Design review of the part built by this model. Coordinates are the model's own, in mm. A direction names the side the tool comes from. Coordinates: 2 decimals unless noted, no trailing zeros. Loops run counter-clockwise (first coordinate to the right, second up) from the corner with the lowest first, then second, coordinate; pieces in that order, holes last.
Q1. Add section B-B on x = -106. Give the boundary of the cut face in (y, z).
Q2. Wall thickness on probe 1 along Z at (x, y) = (-49.5, 190.5); probe 2 along X at (y, z) = (197.5, 81); probe 3 along Z at (x, y) = (-186, 47): over which ranges is each line inside the solid? List them lowest first.
Q3. Add section D-D on y = 19. Give the boundary of the cut face in (x, z).
Q4. Draft analysis for pull direction Y (two halves, no side actions). For faces 5 (the face through (-55.72, 55.49, -4.93)), 6 (the face through (-99, 120, -10)), 7 (the face through (-2.85, 232.99, -22.32)), 8 (the face through (-196.99, 2.85, -22.68)), state which applies: released by +Y, released by -Y, zero draft, split by the parting line, or undercut.
Q5. Add section A-A on y = 190.5. Give the boundary of the cut face in (x, z).
Q6. Machinability: for faces 1 (the face through (-30, 30, 0)), 2 (the face through (-64, 198, 7)), 3 (the face through (-60, 22, -5)), 4 (the face through (-22, 60, -5)), which of the approach directions +Z, -Z, +X, -X, +Y, -Y give a long, thin tool a straight path to every point of the face, cutting with its end or side? Answer none if there is none.
Q7. For P1, Ø3, axis at x = -27, z = -4, coming from the +Y side; P2, Ø8, axis at x = -129, y = 62.5, coming from the +Z side; P3, Ø12, axis at x = -25.5, z = 72, coming from the -Y side, all flat-tipped, find the tip position at first contact; note any pin that passes through.
Q8. Add section C-C on z = 73.5. Give the boundary of the cut face in (x, y), and give its area (3 significant figures).
```python
from build123d import *

# Parameters (mm, degrees)
F1_DEPTH = 200
F0_W     = 60
F0_H     = 10
F2_DEPTH = 60
F0_R     = 20.5
F3_DEPTH = 130
F4_R     = 10
F5_R     = 15


with BuildPart() as f1:
    # F0 (on Right) → F1 (new body)
    with BuildSketch(Plane.YZ):
        Polygon((60, -10), (0, -10), (0, -35), (236, -35), (236, -10), (198, -10), (183, -10), align=None)
    extrude(amount=-F1_DEPTH)

    # F0 (on Right) → F2 (join)
    with BuildSketch(Plane.YZ):
        with Locations((30, -5)):
            Rectangle(F0_W, F0_H)
    extrude(amount=-F2_DEPTH)

    # F0 (on Right) → F3 (join)
    with BuildSketch(Plane.YZ):
        with BuildLine():
            ThreePointArc((226, 60), (168.206503, 87.62698), (183, 25.301297))
            ThreePointArc((183, 25.301297), (190.5, 24.5), (198, 25.301297))
            ThreePointArc((198, 25.301297), (218.12698, 37.706503), (226, 60))
        make_face()
        with Locations((190.5, 60)):
            Circle(F0_R, mode=Mode.SUBTRACT)
        with BuildLine():
            Line((183, 25.301297), (183, -10))
            Line((183, -10), (198, -10))
            Line((198, -10), (198, 25.301297))
            ThreePointArc((198, 25.301297), (190.5, 24.5), (183, 25.301297))
        make_face()
    extrude(amount=-F3_DEPTH)

    # F4
    f4_edges = [f1.edges().sort_by_distance(p)[0] for p in [
        (0, 0, -17.5),
        (-200, 0, -22.5),
        (0, 236, -22.5),
        (-200, 236, -22.5),
    ]]
    fillet(f4_edges, radius=F4_R)

    # F5
    f5_edges = [f1.edges().sort_by_distance(p)[0] for p in [
        (-60, 60, -5),
    ]]
    fillet(f5_edges, radius=F5_R)


solid = f1.part
```
Entries:
1. outline: (0, -35) - (236, -35) - (236, -10) - (198, -10) - (198, 25.3) arc R35.5 ccw to (226, 60) arc R35.5 ccw (long way) to (183, 25.3) - (183, -10) - (0, -10) - close; hole circle Ø41 at (190.5, 60)
2. probe 1: z = -35 to 39.5, 80.5 to 95.5
2. probe 2: x = -130 to 0
2. probe 3: z = -35 to -10
3. outline: (-200, -35) - (0, -35) - (0, 0) - (-60, 0) - (-60, -10) - (-200, -10) - close
4. face 5: undercut
4. face 6: undercut
4. face 7: released by +Y
4. face 8: released by -Y
5. outline: (-200, -35) - (0, -35) - (0, 39.5) - (-130, 39.5) - (-130, -10) - (-200, -10) - close; (-130, 80.5) - (0, 80.5) - (0, 95.5) - (-130, 95.5) - close
6. face 1: +Z, +X, -X, -Y
6. face 2: +X, -X, +Y
6. face 3: +Z, -X, -Y
6. face 4: +Z, +X, -X
7. P1: stops at y = 198
7. P2: stops at z = -10
7. P3: stops at y = 155.51
8. outline: (-130, 157.67) - (0, 157.67) - (0, 175.07) - (-130, 175.07) - close; (-130, 205.93) - (0, 205.93) - (0, 223.33) - (-130, 223.33) - close
8. area: 4,530 mm2
